from build123d import *

# Parameters (mm, degrees)
SKETCH1_R           = 31.75
SKETCH1_R_2         = 2.4765
BOSS_EXTRUDE1_DEPTH = 6.35
SKETCH2_R           = 25.4
CUT_EXTRUDE1_DEPTH  = 1.5875
SKETCH3_R           = 2.4765
BOSS_EXTRUDE2_DEPTH = 6.0452
SKETCH4_R           = 2.54
BOSS_EXTRUDE3_DEPTH = 8.255
CHAMFER1_SIZE       = 0.635
SKETCH5_R           = 6.35
BOSS_EXTRUDE4_DEPTH = 3.302
SKETCH6_R           = 4.445
CUT_EXTRUDE2_DEPTH  = 6.604


with BuildPart() as part:
    # Sketch1 → Boss-Extrude1 (new body)
    with BuildSketch(Plane(origin=(0, 0, 0), x_dir=(1, 0, 0), z_dir=(0, 1, 0))):
        with Locations(Location((0, 0, 0), (0, 0, 270))):
            Circle(SKETCH1_R)
        with Locations(Location((0, 0, 0), (0, 0, 270))):
            Circle(SKETCH1_R_2, mode=Mode.SUBTRACT)
    extrude(amount=BOSS_EXTRUDE1_DEPTH)

    # Sketch2 → Cut-Extrude1 (cut)
    with BuildSketch(Plane(origin=(0, 6.35, 0), x_dir=(1, 0, 0), z_dir=(0, 1, 0))):
        with Locations(Location((0, 0, 0), (0, 0, 270))):
            Circle(SKETCH2_R)
    extrude(amount=-CUT_EXTRUDE1_DEPTH, mode=Mode.SUBTRACT)

    # Sketch3 → Boss-Extrude2 (add)
    with BuildSketch(Plane(origin=(0, 4.7625, 0), x_dir=(1, 0, 0), z_dir=(0, 1, 0))):
        with BuildLine():
            ThreePointArc((-19.002478857, 10.248604651), (0, -21.59), (19.002478857, 10.248604651))
            ThreePointArc((19.002478857, 10.248604651), (0, 6.35), (-19.002478857, 10.248604651))
        make_face()
        with Locations(Location((0, 0, 0), (0, 0, 270))):
            Circle(SKETCH3_R, mode=Mode.SUBTRACT)
    extrude(amount=BOSS_EXTRUDE2_DEPTH)

    # Sketch4 → Boss-Extrude3 (add)
    with BuildSketch(Plane(origin=(0, 6.35, 0), x_dir=(1, 0, 0), z_dir=(0, 1, 0))):
        with Locations(Location((0, 28.575, 0), (0, 0, 270))):
            Circle(SKETCH4_R)
    extrude(amount=BOSS_EXTRUDE3_DEPTH)

    # Chamfer1
    chamfer1_edges = [part.edges().sort_by_distance(p)[0] for p in [
        (0, 14.605, -31.115),
    ]]
    chamfer(chamfer1_edges, length=CHAMFER1_SIZE)

    # Sketch5 → Boss-Extrude4 (add)
    with BuildSketch(Plane.XZ):
        with Locations(Location((0, 0, 0), (0, 0, 90))):
            Circle(SKETCH5_R)
    extrude(amount=BOSS_EXTRUDE4_DEPTH)

    # Sketch6 → Cut-Extrude2 (cut)
    with BuildSketch(Plane.XZ.offset(3.302)):
        with Locations(Location((0, 0, 0), (0, 0, 270))):
            Circle(SKETCH6_R)
    extrude(amount=-CUT_EXTRUDE2_DEPTH, mode=Mode.SUBTRACT)


solid = part.part
Source: CAD feature listing. Evaluate the final solid. Frame: model axes, mm. A direction names the side the tool comes from. Round coordinates to 2 decimals unless told otherwise and drop trailing zeros. Loops run counter-clockwise (first coordinate to the right, second up) from the corner with the lowest first, then second, coordinate; pieces in that order, holes last.
Q1. Section D-D, the plane z = 17. Return loops of the section in (x, y), plus the area to 3 significant figures.
Q2. Ray query, line 1 (X direction, y = 5, z = 0); line 2 (X direction, y = 8, z = 0); line 3 (X direction, y = -0.25, z = 0) (3 decimals). Return the intervals inside material, ascending.
Q3. Mould query, pull axis Z, two halves, no side actions, for faces 4 (the face through (3.86, -1.63, -5.04)), 5 (the face through (0, 4.762, -12)), 6 (the face through (0, 10.808, 5)). Classes: pulls with the +Z half, pulls with the -Z half, needs draft (parallel to the pull), parting line crosses it, or undercut.
Q4. First-contact query: P1, Ø8, axis at x = -7.5, y = 6.5, coming from the +Z side; P2, Ø3, axis at x = 13, z = -5, coming from the +Y side; P3, Ø2, axis at x = 20, y = 7, coming from the +Z side. Flat tips, straight axial feed; report the tip coordinate or a pass-through.
Q5. Access query for faces 1 (the face through (-0.62, 7.74, 21.58)), 2 (the face through (0, 14.605, -29)), 3 (the face through (-4.34, -0.05, 0.96)). Directions: +Z, -Z, +X, -X, +Y, -Y. A direction counts if a zero-diameter tool reaches every point of the face in a straight line with its end or side. Return the directions, or none.
Q6. Section C-C, the plane y = 8.5. Return loops of the section in (x, z) (1 decimal), plus the area to 3 significant figures.
Solutions:
1. outline: (-26.82, 0) - (26.82, 0) - (26.82, 6.35) - (18.87, 6.35) - (18.87, 4.76) - (13.31, 4.76) - (13.31, 10.81) - (-13.31, 10.81) - (-13.31, 4.76) - (-18.87, 4.76) - (-18.87, 6.35) - (-26.82, 6.35) - close
1. area: 442 mm2
2. line 1: x = -31.75 to -25.4, -21.59 to -2.48, 2.48 to 21.59, 25.4 to 31.75
2. line 2: x = -21.59 to -2.48, 2.48 to 21.59
2. line 3: x = -6.35 to -4.445, 4.445 to 6.35
3. face 4: parting line crosses it
3. face 5: undercut
3. face 6: needs draft
4. P1: stops at z = 31.56
4. P2: stops at y = 10.81
4. P3: stops at z = 25.26
5. face 1: +Y
5. face 2: +Z, -Z, +X, -X, +Y
5. face 3: -Y
6. outline: (-19, -10.2) arc R48.3 cw to (19, -10.2) arc R21.6 ccw (long way) to start; circle Ø5.1 at (0, -28.6); hole circle Ø5 at (0, 0)
6. area: 1,060 mm2
